Could you check a few things on this model? Use its own coordinates, in mm. A direction names the side the tool comes from. Give positions to 0.01 mm unless a question says otherwise; leave off trailing zeros. Order: outer loops, then holes, each group sorted by start corner. A loop starts at its lowest first (then second) coordinate and runs counter-clockwise, first axis right, second up. Notation, with made-up numbers: M 18.5,-11 L 56.5,-11 A20 cw 56.5,9 Z; hole C 42.25,43.25 d8. An arc over 180 degrees is marked long. Use a Markdown table: item, result. Add a question column.
```python
from build123d import *

# Parameters (mm, degrees)
SKETCH_1_R      = 1.5
EXTRUDE_1_DEPTH = 0.7
SKETCH_3_R      = 2
EXTRUDE_3_DEPTH = 8
SKETCH_4_R      = 2
EXTRUDE_4_DEPTH = 8


with BuildPart() as part:
    # 草图1 → 凸台-拉伸1 (new body)
    with BuildSketch(Plane(origin=(0, 0, 0), x_dir=(0, 0, -1), z_dir=(1, 0, 0))):
        Polygon((185.963773135, 67.574722086), (185.963773135, 60.574722086), (160.963773135, 60.574722086), (160.963773135, 67.574722086), (160.963773135, 69.848263268), (168.963773135, 69.848263268), (168.963773135, 67.574722086), (177.963773135, 67.574722086), (177.963773135, 69.848263268), (185.963773135, 69.848263268), align=None)
        with Locations((181.963773135, 64.074722086)):
            Circle(SKETCH_1_R, mode=Mode.SUBTRACT)
        with Locations((164.963773135, 64.074722086)):
            Circle(SKETCH_1_R, mode=Mode.SUBTRACT)
    extrude(amount=EXTRUDE_1_DEPTH)

    # 草图3 → 凸台-拉伸3 (add)
    with BuildSketch(Plane.XY.offset(-160.963773135)):
        with Locations((2, 69.848263268)):
            Circle(SKETCH_3_R)
    extrude(amount=-EXTRUDE_3_DEPTH)

    # 草图4 → 凸台-拉伸4 (add)
    with BuildSketch(Plane(origin=(0, 0, -185.963773135), x_dir=(-1, 0, 0), z_dir=(0, 0, -1))):
        with Locations((-2, 69.848263268)):
            Circle(SKETCH_4_R)
    extrude(amount=-EXTRUDE_4_DEPTH)


solid = part.part
```
1) For faces 1 (the face through (0.35, 63.5, -166.35)), 2 (the face through (2, 70, -177.964)), which set-ups out of +Z, -Z, +X, -X, +Y, -Y let a thin tool reach every point of the face, with its end or its side?
2) Please list where these lines run through material, in increasing order: line 1 (Z direction, x = 0.95, y = 70); line 2 (X direction, y = 62, z = -175.5); line 3 (X direction, y = 70, z = -167). Write a range as from..to.
3) Suppose I cut it at C-C on y = 64.5. Please give me the cut outline in (x, z).
4) Suppose I cut it at A-A on x = 2. Please give me the cut outline in (y, z).
5) For pin 1 (4 mm diameter, centred on y = 64.5, z = -169.5, fed in from +X); pin 2 (2.5 mm diameter, centred on y = 64.07, z = -164.96, fed in from -X); pin 3 (0.6 mm diameter, centred on x = 0.5, z = -174.5, fed in from +Y), each with a flat end and sliding along its axis, tell me the tip position at first contact or that it passes through.
6) Suppose I cut it at D-D on z = -177. Please give me the cut outline in (x, y).
7) Suppose I cut it at B-B on z = -182.5. Please give me the cut outline in (x, y).
Values found:
| question | item | result |
|---|---|---|
| 1 | face 1 | +X, -X |
| 1 | face 2 | +X, -X, +Y |
| 2 | line 1 | z = -185.96..-177.96, -168.96..-160.96 |
| 2 | line 2 | x = 0..0.7 |
| 2 | line 3 | x = 0.01..3.99 |
| 3 | outline | M 0,-185.96 L 0.7,-185.96 L 0.7,-183.4 L 0,-183.4 Z; M 0,-180.53 L 0.7,-180.53 L 0.7,-166.4 L 0,-166.4 Z; M 0,-163.53 L 0.7,-163.53 L 0.7,-160.96 L 0,-160.96 Z |
| 4 | outline | M 67.85,-185.96 L 71.85,-185.96 L 71.85,-177.96 L 67.85,-177.96 Z; M 67.85,-168.96 L 71.85,-168.96 L 71.85,-160.96 L 67.85,-160.96 Z |
| 5 | pin 1 | stops at x = 0.7 |
| 5 | pin 2 | passes through |
| 5 | pin 3 | stops at y = 67.57 |
| 6 | outline | M 0,60.57 L 0.7,60.57 L 0.7,67.57 L 0,67.57 Z |
| 7 | outline | M 0,60.57 L 0.7,60.57 L 0.7,62.67 L 0,62.67 Z; M 0,65.48 L 0.7,65.48 L 0.7,68.33 A2 ccw long 0,69.85 Z |
